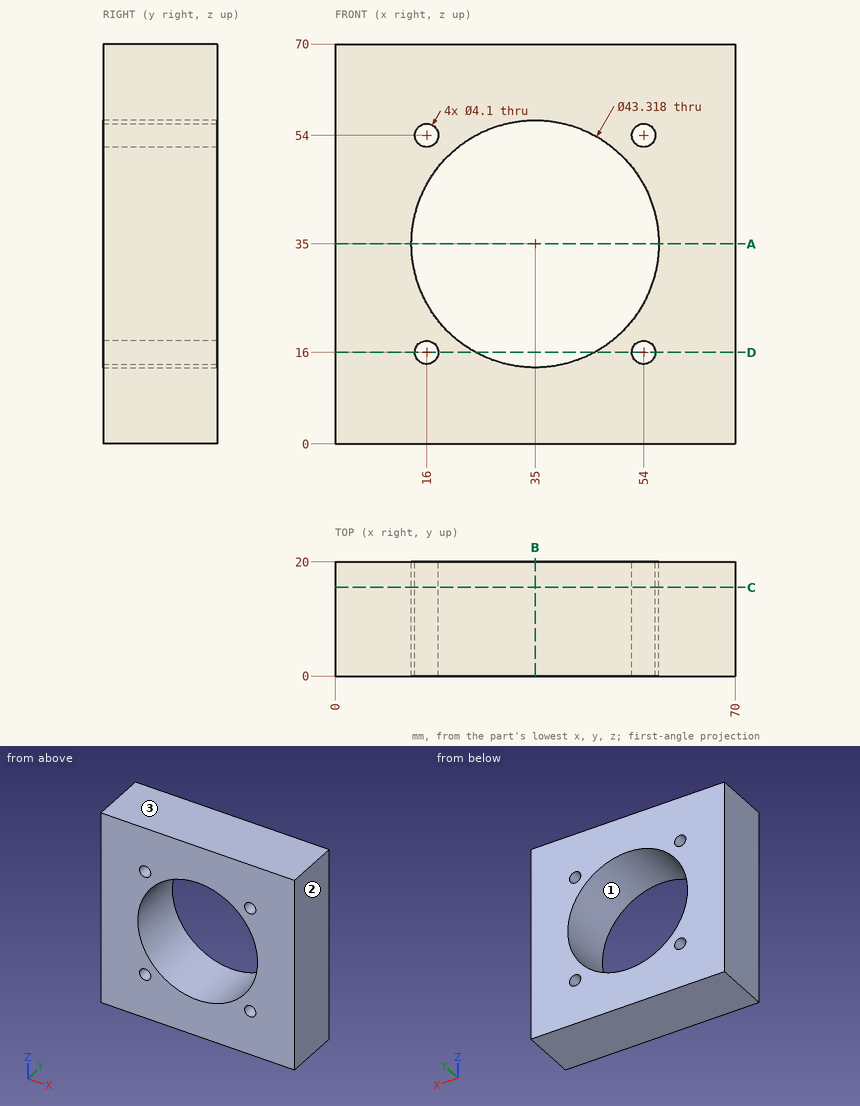
Print and shaded views of the part. All mm, measured from the part's lowest x, y and z. Round coordinates to 2 decimals unless told otherwise and drop trailing zeros. Write each loop counter-clockwise with the first axis right and the second up, starting at its lowest first coordinate (ties: lowest second). Pieces come first, ordered by that corner, then holes. Notation, with made-up numbers: (-36, -5) - (11, -5) arc R16 ccw to (11, 0) - close; hole circle Ø3 at (31.25, 47.5). An arc over 180 degrees is marked (long way). Use CSV: the item, a comma, the result in double quotes. Start each with the question number.
Item 1: Drill centre lines: L1, parallel to X at y = 15.25, z = 55 (1 decimal); L2, parallel to Z at x = 52.5, y = 9.5; L3, parallel to Z at x = 26, y = 19.25. Where is each one in solid material? Low to high. Write a range as [from, to].
Item 2: Band-saw the part on A-A (z = 35). Write the cut outline in (x, y).
Item 3: Band-saw the part on D-D (z = 16). Write the cut outline in (x, y), and give its area (3 significant figures).
Item 4: Two-plate mould, pull along Z, no slides. Class the marked faces 1, 2 and 3: released by +Z, released by -Z, zero draft, split by the parting line, or undercut.
Item 5: Band-saw the part on B-B (x = 35). Write the cut outline in (y, z), and give its area (3 significant figures).
Item 6: Band-saw the part on C-C (y = 15.5). Write the cut outline in (x, z).
Checked values:
1,L1,"x = [0, 14.2], [17.8, 26.7], [43.3, 52.2], [55.8, 70]"
1,L2,"z = [0, 14.6], [17.4, 22.24], [47.76, 52.6], [55.4, 70]"
1,L3,"z = [0, 15.3], [54.7, 70]"
2,outline,"(0, 0) - (13.34, 0) - (13.34, 20) - (0, 20) - close; (56.66, 0) - (70, 0) - (70, 20) - (56.66, 20) - close"
3,outline,"(0, 0) - (13.95, 0) - (13.95, 20) - (0, 20) - close; (18.05, 0) - (24.6, 0) - (24.6, 20) - (18.05, 20) - close; (45.4, 0) - (51.95, 0) - (51.95, 20) - (45.4, 20) - close; (56.05, 0) - (70, 0) - (70, 20) - (56.05, 20) - close"
3,area,"820 mm²"
4,face 1,"undercut"
4,face 2,"zero draft"
4,face 3,"released by +Z"
5,outline,"(0, 0) - (20, 0) - (20, 13.34) - (0, 13.34) - close; (0, 56.66) - (20, 56.66) - (20, 70) - (0, 70) - close"
5,area,"534 mm²"
6,outline,"(0, 0) - (70, 0) - (70, 70) - (0, 70) - close; hole circle Ø43.32 at (35, 35); hole circle Ø4.1 at (16, 16); hole circle Ø4.1 at (16, 54); hole circle Ø4.1 at (54, 16); hole circle Ø4.1 at (54, 54)"
